Verification items for the finished model (mm, model axes). Face numbers are marked on the shaded views. A direction names the side the tool comes from. Coordinates: 2 decimals unless noted, no trailing zeros. Loops run counter-clockwise (first coordinate to the right, second up) from the corner with the lowest first, then second, coordinate; pieces in that order, holes last. Notation, with made-up numbers: M 39.25,-5 L 61.25,-5 A9 cw 61.25,4 Z; hole C -35.5,50.5 d5. An arc over 180 degrees is marked long. Write item = value, one per line. Start each with the question number.
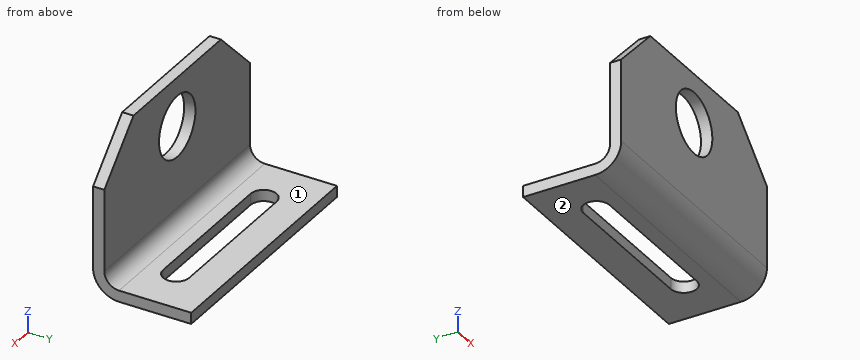
```python
from build123d import *

# Parameters (mm, degrees)
F1_DEPTH      = 25
F1_DEPTH_BACK = 25
F4_DEPTH      = 2.301
F5_R          = 3
F6_R          = 5.3
F7_D          = 12.5
F8_SIZE       = 10


with BuildPart() as f1:
    # F0 (on Right) → F1 (new body, two sides)
    with BuildSketch(Plane.YZ) as f1_sk:
        Polygon((2.3, 32), (0, 32), (0, 0), (20, 0), (20, 2.3), (2.3, 2.3), align=None)
    extrude(amount=F1_DEPTH)
    extrude(f1_sk.sketch, amount=-F1_DEPTH_BACK)

    # F3 (on face) → F4 (cut, through all)
    with BuildSketch(Plane.XY.offset(2.3)):
        with BuildLine():
            Line((-15, 8.35), (15, 8.35))
            ThreePointArc((15, 8.35), (17.65, 11), (15, 13.65))
            Line((15, 13.65), (-15, 13.65))
            ThreePointArc((-15, 13.65), (-17.65, 11), (-15, 8.35))
        make_face()
    extrude(amount=-F4_DEPTH, mode=Mode.SUBTRACT)

    # F5
    f5_edges = [f1.edges().sort_by_distance(p)[0] for p in [
        (0, 2.3, 2.3),
    ]]
    fillet(f5_edges, radius=F5_R)

    # F6
    f6_edges = [f1.edges().sort_by_distance(p)[0] for p in [
        (0, 0, 0),
    ]]
    fillet(f6_edges, radius=F6_R)

    # F7 (through all)
    with Locations(Plane.XZ):
        with Locations((0, 22)):
            Hole(F7_D / 2)

    # F8
    f8_edges = [f1.edges().sort_by_distance(p)[0] for p in [
        (25, 1.15, 32),
        (-25, 1.15, 32),
    ]]
    chamfer(f8_edges, length=F8_SIZE)


solid = f1.part
```
Q1. Sectioned sample at A-A on x = 0. Record the cut outline in (y, z).
Q2. Sectioned sample at D-D on x = 8.5. Record the cut outline in (y, z), plus the area to 3 significant figures.
Q3. Sectioned sample at B-B on z = 17. Record the cut outline in (x, y).
Q4. Gauge pin test, flat ends, axial feed: pin 1 (2.5 mm diameter, centred on x = -4.5, z = 1.5, fed in from -Y); pin 2 (10 mm diameter, centred on x = -15.5, y = 14, fed in from +Z); pin 3 (7.5 mm diameter, centred on x = 0, z = 22, fed in from -Y). Record the tip position at first contact, or that the pin passes through.
Q5. Sectioned sample at C-C on y = 11. Record the cut outline in (x, z), plus the area to 3 significant figures.
Q6. Scan lines: L1, parallel to Z at x = 20, y = 10; L2, parallel to X at y = 1.75, z = 17. Record each from-to range of solid material in increasing order. Write a range as [from, to].
Q7. Set-up check for the marked faces 1 and 2: record each of +Z, -Z, +X, -X, +Y, -Y from which the full face is reachable in a straight line by a thin tool's end or side.
Solutions:
q1.outline = M 0,5.3 A5.3 ccw 5.3,0 L 8.35,0 L 8.35,2.3 L 5.3,2.3 A3 cw 2.3,5.3 L 2.3,15.75 L 0,15.75 Z; M 0,28.25 L 2.3,28.25 L 2.3,32 L 0,32 Z; M 13.65,0 L 20,0 L 20,2.3 L 13.65,2.3 Z
q2.outline = M 0,5.3 A5.3 ccw 5.3,0 L 8.35,0 L 8.35,2.3 L 5.3,2.3 A3 cw 2.3,5.3 L 2.3,32 L 0,32 Z; M 13.65,0 L 20,0 L 20,2.3 L 13.65,2.3 Z
q2.area = 98.0 mm²
q3.outline = M -25,0 L -3.75,0 L -3.75,2.3 L -25,2.3 Z; M 3.75,0 L 25,0 L 25,2.3 L 3.75,2.3 Z
q4.pin_1 = 0.65
q4.pin_2 = 2.3
q4.pin_3 = through
q5.outline = M -25,0 L -17.65,0 L -17.65,2.3 L -25,2.3 Z; M 17.65,0 L 25,0 L 25,2.3 L 17.65,2.3 Z
q5.area = 33.8 mm²
q6.L1 = [0, 2.3]
q6.L2 = [-25, -3.75], [3.75, 25]
q7.face_1 = +Z, +X, -X, +Y
q7.face_2 = -Z, +X, -X, +Y, -Y
